```python
from build123d import *

# Parameters (mm, degrees)
F0_R     = 3.5
F1_DEPTH = 4
F0_R_2   = 1.75
F2_DEPTH = 4
F3_SIZE  = 1.78
F4_DEPTH = 2


# Not quite as in the source:
# - a feature names something its author has since deleted; it is built from what else it names


with BuildPart() as f1:
    # F0 (on Top) → F1 (new body)
    with BuildSketch(Plane.XY):
        Polygon((0, 44.6608208763), (0, 0), (19, 0), (32.9255871796, 14.3554178519), (10, 44.6608208763), align=None)
        with Locations((9.5, 6)):
            Circle(F0_R, mode=Mode.SUBTRACT)
        with Locations((15.8802193485, 25.2849848836)):
            Circle(F0_R, mode=Mode.SUBTRACT)
        Polygon((-9.5, 0), (0, 0), (0, 44.6608208763), (-10, 44.6608208763), (-32.9255871796, 14.3554178519), (-19, 0), align=None)
        with Locations((-9.5, 6)):
            Circle(F0_R, mode=Mode.SUBTRACT)
        with Locations((-15.8802193485, 25.2849848836)):
            Circle(F0_R, mode=Mode.SUBTRACT)
    extrude(amount=F1_DEPTH)

    # F0 (on Top) → F2 (join)
    with BuildSketch(Plane.XY):
        with Locations((9.5, 6)):
            Circle(F0_R)
        with Locations((9.5, 6)):
            Circle(F0_R_2, mode=Mode.SUBTRACT)
        with Locations((-9.5, 6)):
            Circle(F0_R)
        with Locations((-9.5, 6)):
            Circle(F0_R_2, mode=Mode.SUBTRACT)
        with Locations((-15.8802193485, 25.2849848836)):
            Circle(F0_R)
        with Locations((-15.8802193485, 25.2849848836)):
            Circle(F0_R_2, mode=Mode.SUBTRACT)
        with Locations((15.8802193485, 25.2849848836)):
            Circle(F0_R)
        with Locations((15.8802193485, 25.2849848836)):
            Circle(F0_R_2, mode=Mode.SUBTRACT)
    extrude(amount=F2_DEPTH)

    # F3
    f3_edges = [f1.edges().sort_by_distance(p)[0] for p in [
        (14.130219, 25.284985, 4),
        (-17.630219, 25.284985, 4),
        (-11.25, 6, 4),
        (7.75, 6, 4),
    ]]
    chamfer(f3_edges, length=F3_SIZE)

    # F0 (on Top) → F4 (cut)
    with BuildSketch(Plane.XY):
        with Locations((-15.8802193485, 25.2849848836)):
            Circle(F0_R)
        with Locations((-15.8802193485, 25.2849848836)):
            Circle(F0_R_2, mode=Mode.SUBTRACT)
        with Locations((15.8802193485, 25.2849848836)):
            Circle(F0_R)
        with Locations((15.8802193485, 25.2849848836)):
            Circle(F0_R_2, mode=Mode.SUBTRACT)
        with Locations((9.5, 6)):
            Circle(F0_R)
        with Locations((9.5, 6)):
            Circle(F0_R_2, mode=Mode.SUBTRACT)
        with Locations((-9.5, 6)):
            Circle(F0_R)
        with Locations((-9.5, 6)):
            Circle(F0_R_2, mode=Mode.SUBTRACT)
    extrude(amount=F4_DEPTH, mode=Mode.SUBTRACT)


solid = f1.part
```
The listing builds one solid part. Answer for the finished solid, in the listing's coordinates (mm). A direction names the side the tool comes from. Round coordinates to 2 decimals unless told otherwise and drop trailing zeros. Loops run counter-clockwise (first coordinate to the right, second up) from the corner with the lowest first, then second, coordinate; pieces in that order, holes last. Notation, with made-up numbers: (44.5, 21) - (100.5, 21) arc R18 cw to (100.5, 54) - close; hole circle Ø1 at (65, -14.75). An arc over 180 degrees is marked (long way). Use one line per item in the form item = value. Start each with the question number.
1. A tool of negligible diameter and unlimited length cuts with its end or side. For faces 4 (the face through (25.87, 7.08, 1.97)), 5 (the face through (19.219, 26.336, 0.986)), from which of +Z, -Z, +X, -X, +Y, -Y can it reach the whole face along a straight path? Write none if from no direction.
2. For a pull along X with two mould halves and no side action, classify faces 1 (the face through (0, 23, 4)), 2 (the face through (-21.302, 29.72, 1.972)), 3 (the face through (-15, 27, 2)) as pulls with the +X half, pulls with the -X half, needs draft (parallel to the pull), parting line crosses it, or undercut.
3. The part is cut by section B-B on y = 6. Determine the outline of the cut face in (x, z), then the cut area to 3 significant figures.
4. The part is cut by section C-C on x = -22. Determine the outline of the cut face in (y, z).
5. The part is cut by section D-D on y = 24.5. Give the number of separate pieces and of enclosed holes in the cut face, then the cut area to 3 significant figures.
6. Given pin 1 Ø3.5 at (x, y) = (-15.5, 25.5) entering from -Z; pin 2 Ø5 at (x, y) = (9, 26.5) entering from -Z; pin 3 Ø3 at (x, y) = (-15.88, 25.28) entering from +Z; pin 4 Ø4.5 at (x, y) = (9.5, 6) entering from +Z, each flat-ended and moving along its own axis, determine where each tip first touches the part or whether it passes through.
7. Consider line 1 (X direction, y = 3, z = 1.7); line 2 (X direction, y = 7, z = 3.1); line 3 (Y direction, x = -9.5, z = 2.1). Determine where each line is inside the solid, lowest interval first. Write a range as [from, to].
8. The part is cut by section A-A on z = 3.1. Determine the outline of the cut face in (x, y).
Geometry check:
q1.face_4 = +Z, -Z, +X, -Y
q1.face_5 = -Z
q2.face_1 = needs draft
q2.face_2 = pulls with the -X half
q2.face_3 = undercut
q3.outline = (-24.82, 0) - (-13, 0) - (-13, 2) - (-11.25, 2) - (-11.25, 2.22) - (-13.03, 4) - (-24.82, 4) - close; (-7.75, 2) - (-6, 2) - (-6, 0) - (6, 0) - (6, 2) - (7.75, 2) - (7.75, 2.22) - (5.97, 4) - (-5.97, 4) - (-7.75, 2.22) - close; (11.25, 2) - (13, 2) - (13, 0) - (24.82, 0) - (24.82, 4) - (13.03, 4) - (11.25, 2.22) - close
q3.area = 150 mm^2
q4.outline = (3.09, 0) - (28.8, 0) - (28.8, 4) - (3.09, 4) - close
q5.separate_pieces = 3
q5.enclosed_holes = 0
q5.area = 155 mm^2
q6.pin_1 = 2
q6.pin_2 = 0
q6.pin_3 = through
q6.pin_4 = 2.72
q7.line_1 = [-21.91, -11.3], [-7.7, 7.7], [11.3, 21.91]
q7.line_2 = [-25.79, -11.93], [-7.07, 7.07], [11.93, 25.79]
q7.line_3 = [0, 4.25], [7.75, 44.66]
q8.outline = (-32.93, 14.36) - (-19, 0) - (19, 0) - (32.93, 14.36) - (10, 44.66) - (-10, 44.66) - close; hole circle Ø5.26 at (-15.88, 25.28); hole circle Ø5.26 at (-9.5, 6); hole circle Ø5.26 at (9.5, 6); hole circle Ø5.26 at (15.88, 25.28)
